Work out the finished part from the listing and answer in its coordinate system (mm). A direction names the side the tool comes from. Coordinates: 2 decimals unless noted, no trailing zeros. Order: outer loops, then holes, each group sorted by start corner. A loop starts at its lowest first (then second) coordinate and runs counter-clockwise, first axis right, second up. Notation, with made-up numbers: (-18, -5) -> (23, -5) arc R25 cw to (23, 28) -> close; hole circle Ø6 at (-15, -24.5). An arc over 180 degrees is marked (long way). Write item = value, one per line. Start each with the question number.
Q1. For a pull along Y with two mould halves and no side action, classify faces 1 (the cylindrical face through (-5.69, 32.01, -5.16)), 2 (the flat face through (-6, 22, -15.2)), 3 (the flat face through (-6, 55, -6)), 4 (the flat face through (-5, 27, 6)) as +Y half, -Y half, draft (parallel to the pull), parting line (faces both ways), or undercut.
Q2. The part is cut by section D-D, the plane x = -13. Determine the outline of the cut face in (y, z), plus the area to 3 significant figures.
Q3. The part is cut by section B-B, the plane x = -2.5. Determine the outline of the cut face in (y, z), plus the area to 3 significant figures.
Q4. Straight lines are drawn through the part: L1, parallel to Z at x = -8, y = 42; L2, parallel to X at y = 7, z = -3; L3, parallel to Y at x = -9.5, z = 2.75. For each, find the intervals that lie inside material, in ascending order. Write a range as from..to.
Q5. Flat-ended cylindrical pins translate along their axes: pin 1 (3 mm diameter, centred on y = 7.5, z = 1, fed in from -X); pin 2 (6 mm diameter, centred on y = 45.5, z = -13, fed in from +X); pin 3 (9.5 mm diameter, centred on x = -6.5, y = 7.5, fed in from +Z). Find the tip coordinate at first contact, or state that the pin passes through.
Q6. Which of the six approach directions +Z, -Z, +X, -X, +Y, -Y give full straight-line access (tool end or side, diameter ignored) to faces 5 (the cylindrical face through (-13.87, 21.91, 3.41)), 6 (the flat face through (-6, 20, -12)), 7 (the flat face through (-0.1, 11, -6)), 8 (the flat face through (-6, 22, 4))?
Q7. The part is cut by section C-C, the plane y = 15.5. Determine the outline of the cut face in (x, z).
Q8. The part is cut by section A-A, the plane y = 42. Determine the outline of the cut face in (x, z) (3 decimals), plus the area to 3 significant figures.
```python
from build123d import *

# Parameters (mm, degrees)
SKETCH1_W           = 35
SKETCH1_H           = 27.2
BOSS_EXTRUDE1_DEPTH = 19.2
SKETCH2_W           = 4
SKETCH2_H           = 5
CUT_EXTRUDE1_DEPTH  = 20.2
SKETCH3_W           = 4
SKETCH3_H           = 5
CUT_EXTRUDE2_DEPTH  = 20.2
SKETCH4_W           = 11
SKETCH4_H           = 11
BOSS_EXTRUDE2_DEPTH = 20
DRAFT1_ANGLE        = 45
DRAFT2_ANGLE        = 45
FILLET1_R           = 1.27
FILLET2_R           = 3.175
FILLET3_R           = 10


with BuildPart() as part:
    # Sketch1 → Boss-Extrude1 (new body)
    with BuildSketch(Plane(origin=(-15.2, 0, 0), x_dir=(0, -1, 0), z_dir=(-1, 0, 0))):
        with Locations((-37.5, -5.6)):
            Rectangle(SKETCH1_W, SKETCH1_H)
    extrude(amount=-BOSS_EXTRUDE1_DEPTH)

    # Sketch2 → Cut-Extrude1 (cut, through all)
    with BuildSketch(Plane(origin=(4, 0, 0), x_dir=(0, 0, -1), z_dir=(1, 0, 0))):
        with Locations((-6, 22.5)):
            Rectangle(SKETCH2_W, SKETCH2_H)
    extrude(amount=-CUT_EXTRUDE1_DEPTH, mode=Mode.SUBTRACT)

    # Sketch3 → Cut-Extrude2 (cut, through all)
    with BuildSketch(Plane(origin=(4, 0, 0), x_dir=(0, 0, -1), z_dir=(1, 0, 0))):
        with Locations((17.2, 22.5)):
            Rectangle(SKETCH3_W, SKETCH3_H)
    extrude(amount=-CUT_EXTRUDE2_DEPTH, mode=Mode.SUBTRACT)

    # Sketch4 → Boss-Extrude2 (add)
    with BuildSketch(Plane.XZ.offset(-20)):
        with Locations((-5.6, -5.6)):
            Rectangle(SKETCH4_W, SKETCH4_H)
    extrude(amount=BOSS_EXTRUDE2_DEPTH)

    # Draft1
    draft1_faces = [part.faces().sort_by_distance(p)[0] for p in [
        (-5.6, 25, 6),
    ]]
    draft(draft1_faces, Plane(origin=(-15.2, 20, 4), x_dir=(1, 0, 0), z_dir=(0, 0, 1)), DRAFT1_ANGLE)

    # Draft2
    draft2_faces = [part.faces().sort_by_distance(p)[0] for p in [
        (-5.6, 25, -17.2),
    ]]
    draft(draft2_faces, Plane(origin=(-15.2, 25, -15.2), x_dir=(0, -1, 0), z_dir=(0, 0, -1)), DRAFT2_ANGLE)

    # Sketch5 → Cut-Revolve1 (revolve, cut)
    with BuildSketch(Plane.XY.offset(-5.6)):
        with BuildLine():
            Line((-15.2, 55.175), (-15.2, 42))
            Line((-15.2, 42), (4, 42))
            Line((4, 42), (4, 55.175))
            ThreePointArc((4, 55.175), (3.07006403, 52.92993597), (0.825, 52))
            Line((0.825, 52), (-12.025, 52))
            ThreePointArc((-12.025, 52), (-14.27006403, 52.92993597), (-15.2, 55.175))
        make_face()
    revolve(axis=Axis((-15.2, 42, -5.6), (1, 0, 0)), mode=Mode.SUBTRACT)

    # Fillet1
    fillet1_edges = [part.edges().sort_by_distance(p)[0] for p in [
        (-0.1, 10, -11.1),
        (-0.1, 10, -0.1),
        (-11.1, 10, -0.1),
        (-11.1, 10, -11.1),
        (-0.1, 0, -5.6),
        (-5.6, 0, -0.1),
        (-11.1, 0, -5.6),
        (-5.6, 0, -11.1),
    ]]
    fillet(fillet1_edges, radius=FILLET1_R)

    # Fillet2
    fillet2_edges = [part.edges().sort_by_distance(p)[0] for p in [
        (-15.2, 22.5, 4),
        (4, 22.5, 4),
        (-15.2, 22.5, -15.2),
        (4, 22.5, -15.2),
    ]]
    fillet(fillet2_edges, radius=FILLET2_R)

    # Fillet3
    fillet3_edges = [part.edges().sort_by_distance(p)[0] for p in [
        (-5.6, 55, 8),
        (-5.6, 55, -19.2),
    ]]
    fillet(fillet3_edges, radius=FILLET3_R)


solid = part.part
```
Model answer:
q1.face_1 = undercut
q1.face_2 = draft
q1.face_3 = +Y half
q1.face_4 = -Y half
q2.outline = (20, -15.05) -> (24.85, -15.05) -> (29, -19.2) -> (45, -19.2) arc R10 ccw to (55, -9.2) -> (55, -2) arc R10 ccw to (45, 8) -> (29, 8) -> (24.85, 3.85) -> (20, 3.85) -> close; hole circle Ø20.31 at (42, -5.6)
q2.area = 528 mm2
q3.outline = (0, -9.83) arc R1.27 ccw to (1.27, -11.1) -> (20, -11.1) -> (20, -15.2) -> (25, -15.2) -> (29, -19.2) -> (45, -19.2) arc R10 ccw to (55, -9.2) -> (55, -2) arc R10 ccw to (45, 8) -> (29, 8) -> (25, 4) -> (20, 4) -> (20, -0.1) -> (1.27, -0.1) arc R1.27 ccw to (0, -1.37) -> close; hole circle Ø20 at (42, -5.6)
q3.area = 758 mm2
q4.L1 = -19.2..-15.6, 4.4..8
q4.L2 = -11.1..-0.1
q4.L3 = 20..36.5, 47.5..53.8
q5.pin_1 = -10.76
q5.pin_2 = 3.3
q5.pin_3 = -0.1
q6.face_5 = +Z, -X, -Y
q6.face_6 = -Y
q6.face_7 = +Z, -Z, +X, -Y
q6.face_8 = +Z, +X, -X, -Y
q7.outline = (-11.1, -9.83) arc R1.27 ccw to (-9.83, -11.1) -> (-1.37, -11.1) arc R1.27 ccw to (-0.1, -9.83) -> (-0.1, -1.37) arc R1.27 ccw to (-1.37, -0.1) -> (-9.83, -0.1) arc R1.27 ccw to (-11.1, -1.37) -> close
q8.outline = (-15.2, -19.2) -> (4, -19.2) -> (4, -18.775) arc R3.175 ccw to (0.825, -15.6) -> (-12.025, -15.6) arc R3.175 ccw to (-15.2, -18.775) -> close; (-15.2, 7.575) arc R3.175 ccw to (-12.025, 4.4) -> (0.825, 4.4) arc R3.175 ccw to (4, 7.575) -> (4, 8) -> (-15.2, 8) -> close
q8.area = 130 mm2
